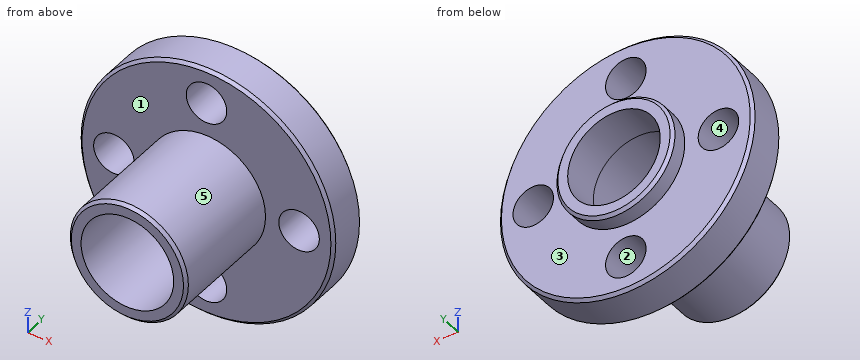
from build123d import *

# Parameters (mm, degrees)
SKETCH1_R                = 11
SKETCH1_R_2              = 5.1
SKETCH1_R_3              = 1.75
BOSS_EXTRUDE1_DEPTH      = 1.75
SKETCH1_3_R              = 5.1
SKETCH1_3_R_2            = 4
BOSS_EXTRUDE2_DEPTH      = 3.25
BOSS_EXTRUDE2_DEPTH_BACK = 11.75
CHAMFER1_SIZE            = 0.25


with BuildPart() as part:
    # Sketch1 → Boss-Extrude1 (new body, symmetric)
    with BuildSketch(Plane(origin=(0, 0, 0), x_dir=(1, 0, 0), z_dir=(0, 1, 0))):
        Circle(SKETCH1_R)
        Circle(SKETCH1_R_2, mode=Mode.SUBTRACT)
        with Locations((0, 8)):
            Circle(SKETCH1_R_3, mode=Mode.SUBTRACT)
        with Locations((8, 0)):
            Circle(SKETCH1_R_3, mode=Mode.SUBTRACT)
        with Locations((0, -8)):
            Circle(SKETCH1_R_3, mode=Mode.SUBTRACT)
        with Locations((-8, 0)):
            Circle(SKETCH1_R_3, mode=Mode.SUBTRACT)
    extrude(amount=BOSS_EXTRUDE1_DEPTH, both=True)

    # Sketch1_3 → Boss-Extrude2 (add, two sides)
    with BuildSketch(Plane(origin=(0, 0, 0), x_dir=(1, 0, 0), z_dir=(0, 1, 0))) as boss_extrude2_sk:
        Circle(SKETCH1_3_R)
        Circle(SKETCH1_3_R_2, mode=Mode.SUBTRACT)
    extrude(amount=BOSS_EXTRUDE2_DEPTH)
    extrude(boss_extrude2_sk.sketch, amount=-BOSS_EXTRUDE2_DEPTH_BACK)

    # Chamfer1
    chamfer1_edges = [part.edges().sort_by_distance(p)[0] for p in [
        (-11, -1.75, 0),
        (-5.1, -11.75, 0),
        (-5.1, 3.25, 0),
        (-11, 1.75, 0),
    ]]
    chamfer(chamfer1_edges, length=CHAMFER1_SIZE)


solid = part.part
CAD build for the part. Positions are in the model's coordinates, mm. Face numbers are marked on the shaded views. A direction names the side the tool comes from. Coordinates: 2 decimals unless noted, no trailing zeros. Write each loop counter-clockwise with the first axis right and the second up, starting at its lowest first coordinate (ties: lowest second). Pieces come first, ordered by that corner, then holes. Notation, with made-up numbers: M 38.25,31.25 L 87.25,31.25 A23 ccw 87.25,44.25 Z; hole C 71.25,42.5 d6. An arc over 180 degrees is marked long. Answer as a JSON object with one key per item and string values. Group by question number.
1) Saw through at A-A (x = 0). Give the number of separate pieces and of enclosed holes in the cut face, plus the area to 4 significant figures.
2) Wall check: line 1 (X direction, y = -0.05, z = 0); line 2 (X direction, y = -8.75, z = 0). Give the ranges that are in metal, low to high. Write a range as from..to.
3) Tool access for the marked faces 1 and 2: list every direction of +Z, -Z, +X, -X, +Y, -Y with a clear straight run to the whole face (end or side of a thin tool).
4) Mould opens along Z. For the marked faces 3, 4 and 5 say: +Z half, -Z half, draft (parallel to the pull), parting line (faces both ways), or undercut.
5) Pin check, flat tips, straight feed: pin 1 Ø6 at (y, z) = (1, -8.5) entering from -X; pin 2 Ø1 at (x, y) = (3.5, -2.5) entering from +Z; pin 3 Ø9 at (x, z) = (0, 0) entering from -Y; pin 4 Ø1 at (x, z) = (5.5, 4) entering from +Y. Stop position of each tip, or through.
6) Saw through at C-C (y = -8). Write the cut outline in (x, z).
Values follow:
{
 "1": {"separate pieces": "4", "enclosed holes": "0", "area": "49.55 mm2"},
 "2": {"line 1": "x = -11..-9.75, -6.25..-4, 4..6.25, 9.75..11", "line 2": "x = -5.1..-4, 4..5.1"},
 "3": {"face 1": "-Y", "face 2": "+Y, -Y"},
 "4": {"face 3": "draft", "face 4": "undercut", "face 5": "parting line"},
 "5": {"pin 1": "stops at x = -9.53", "pin 2": "stops at z = 4.12", "pin 3": "stops at y = -11.75", "pin 4": "stops at y = 1.75"},
 "6": {"outline": "C 0,0 d10.2; hole C 0,0 d8"}
}
